The model under review builds one solid part; all positions refer to its coordinate system, in mm. Face numbers are marked on the shaded views. A direction names the side the tool comes from. Coordinates: 2 decimals unless noted, no trailing zeros. Loops run counter-clockwise (first coordinate to the right, second up) from the corner with the lowest first, then second, coordinate; pieces in that order, holes last. Notation, with made-up numbers: (-24, -28.75) - (-16, -28.75) arc R17 ccw to (-16, 3.25) - close; hole circle Ø8 at (63.25, -25.5). An arc over 180 degrees is marked (long way). Answer in a Markdown table with one row per item. Add a question column.
(1) For P1, Ø5, axis at x = 6.5, z = 6.5, coming from the -Y side; P2, Ø0.8, axis at x = -2, z = 4.5, coming from the +Y side; P3, Ø0.5, axis at x = 1.5, z = 4, coming from the -Y side, all flat-tipped, find the tip position at first contact; note any pin that passes through.
(2) Machinability: for the marked faces 1, 2, 3, 4 and 5, which of the approach directions +Z, -Z, +X, -X, +Y, -Y give a long, thin tool a straight path to every point of the face, cutting with its end or side? Answer none if there is none.
(3) We need section D-D on z = 9.25. Write out the cut boundary in (x, y), plus the area to 3 significant figures.
(4) For line 1 along X through (y, z) = (0.25, 8); line 2 along X through (y, z) = (0.25, 0.25); line 3 along Z through (x, y) = (1.5, 7), list the stretches that pass through material, from the lowest coordinate up.
(5) We need section B-B on y = 0. Write out the cut boundary in (x, z) (1 decimal), plus the area to 3 significant figures.
(6) We need section A-A on z = -4.5. Write out the cut boundary in (x, y).
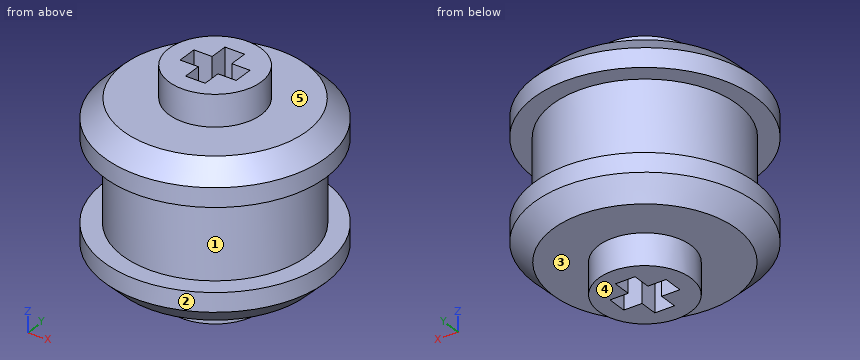
from build123d import *

# Parameters (mm, degrees)
F0_R      = 7.9375
F1_DEPTH  = 7
F2_R      = 9.525
F2_R_2    = 7.9375
F3_DEPTH  = 3.2512
F4_R      = 9.525
F4_R_2    = 7.9375
F5_DEPTH  = 3.2512
F6_SIZE   = 1.6256
F7_R      = 3.96875
F8_DEPTH  = 2.6975943
F9_R      = 3.96875
F10_DEPTH = 2.6975943


with BuildPart() as f1:
    # F0 (on Top) → F1 (new body)
    with BuildSketch(Plane.XY):
        Circle(F0_R)
        Polygon((0.84455, 0.84455), (2.413, 0.84455), (2.413, -0.84455), (0.84455, -0.84455), (0.84455, -2.413), (-0.84455, -2.413), (-0.84455, -0.84455), (-2.413, -0.84455), (-2.413, 0.84455), (-0.84455, 0.84455), (-0.84455, 2.413), (0.84455, 2.413), align=None, mode=Mode.SUBTRACT)
    extrude(amount=F1_DEPTH)

    # F2 (on face) → F3 (join)
    with BuildSketch(Plane.XY.offset(7)):
        Circle(F2_R)
        Circle(F2_R_2, mode=Mode.SUBTRACT)
        Circle(F2_R_2)
        Polygon((0.84455, 2.413), (0.84455, 0.84455), (2.413, 0.84455), (2.413, -0.84455), (0.84455, -0.84455), (0.84455, -2.413), (-0.84455, -2.413), (-0.84455, -0.84455), (-2.413, -0.84455), (-2.413, 0.84455), (-0.84455, 0.84455), (-0.84455, 2.413), align=None, mode=Mode.SUBTRACT)
    extrude(amount=F3_DEPTH)

    # F4 (on face) → F5 (join)
    with BuildSketch(Plane(origin=(0, 0, 0), x_dir=(1, 0, 0), z_dir=(0, 0, -1))):
        Circle(F4_R)
        Circle(F4_R_2, mode=Mode.SUBTRACT)
        Circle(F4_R_2)
        Polygon((2.413, 0.84455), (2.413, -0.84455), (0.84455, -0.84455), (0.84455, -2.413), (-0.84455, -2.413), (-0.84455, -0.84455), (-2.413, -0.84455), (-2.413, 0.84455), (-0.84455, 0.84455), (-0.84455, 2.413), (0.84455, 2.413), (0.84455, 0.84455), align=None, mode=Mode.SUBTRACT)
    extrude(amount=F5_DEPTH)

    # F6
    f6_edges = [f1.edges().sort_by_distance(p)[0] for p in [
        (-9.525, 0, 10.2512),
        (-9.525, 0, -3.2512),
    ]]
    chamfer(f6_edges, length=F6_SIZE)

    # F7 (on face) → F8 (join)
    with BuildSketch(Plane.XY.offset(10.2512)):
        Circle(F7_R)
        Polygon((-2.413, -0.84455), (-2.413, 0.84455), (-0.84455, 0.84455), (-0.84455, 2.413), (0.84455, 2.413), (0.84455, 0.84455), (2.413, 0.84455), (2.413, -0.84455), (0.84455, -0.84455), (0.84455, -2.413), (-0.84455, -2.413), (-0.84455, -0.84455), align=None, mode=Mode.SUBTRACT)
    extrude(amount=F8_DEPTH)

    # F9 (on face) → F10 (join)
    with BuildSketch(Plane(origin=(0, 0, -3.2512), x_dir=(1, 0, 0), z_dir=(0, 0, -1))):
        Circle(F9_R)
        Polygon((-0.84455, 2.413), (0.84455, 2.413), (0.84455, 0.84455), (2.413, 0.84455), (2.413, -0.84455), (0.84455, -0.84455), (0.84455, -2.413), (-0.84455, -2.413), (-0.84455, -0.84455), (-2.413, -0.84455), (-2.413, 0.84455), (-0.84455, 0.84455), align=None, mode=Mode.SUBTRACT)
    extrude(amount=F10_DEPTH)


solid = f1.part
Outcome:
| question | item | result |
|---|---|---|
| 1 | P1 | y = -8.62 |
| 1 | P2 | y = 7.77 |
| 1 | P3 | y = -7.84 |
| 2 | face 1 | none |
| 2 | face 2 | +Z, -Z |
| 2 | face 3 | -Z |
| 2 | face 4 | -Z, +X, -X, +Y, -Y |
| 2 | face 5 | +Z |
| 3 | outline | circle Ø17.8 at (0, 0); hole (-2.41, -0.84) - (-0.84, -0.84) - (-0.84, -2.41) - (0.84, -2.41) - (0.84, -0.84) - (2.41, -0.84) - (2.41, 0.84) - (0.84, 0.84) - (0.84, 2.41) - (-0.84, 2.41) - (-0.84, 0.84) - (-2.41, 0.84) - close |
| 3 | area | 235 mm² |
| 4 | line 1 | -9.52 to -2.41, 2.41 to 9.52 |
| 4 | line 2 | -7.93 to -2.41, 2.41 to 7.93 |
| 4 | line 3 | -3.25 to 10.25 |
| 5 | outline | (-9.5, -1.6) - (-7.9, -3.3) - (-4, -3.3) - (-4, -5.9) - (-2.4, -5.9) - (-2.4, 12.9) - (-4, 12.9) - (-4, 10.3) - (-7.9, 10.3) - (-9.5, 8.6) - (-9.5, 7) - (-7.9, 7) - (-7.9, 0) - (-9.5, 0) - close; (2.4, -5.9) - (4, -5.9) - (4, -3.3) - (7.9, -3.3) - (9.5, -1.6) - (9.5, 0) - (7.9, 0) - (7.9, 7) - (9.5, 7) - (9.5, 8.6) - (7.9, 10.3) - (4, 10.3) - (4, 12.9) - (2.4, 12.9) - close |
| 5 | area | 181 mm² |
| 6 | outline | circle Ø7.94 at (0, 0); hole (-2.41, -0.84) - (-0.84, -0.84) - (-0.84, -2.41) - (0.84, -2.41) - (0.84, -0.84) - (2.41, -0.84) - (2.41, 0.84) - (0.84, 0.84) - (0.84, 2.41) - (-0.84, 2.41) - (-0.84, 0.84) - (-2.41, 0.84) - close |
